Input: dimensioned drawing with shaded views. Units: mm. Origin: part minimum x, y, z. Give positions to 0.01 mm unless a question says otherwise; leave off trailing zeros. Write each loop counter-clockwise with the first axis right and the second up, starting at its lowest first coordinate (ties: lowest second). Pieces come first, ordered by that corner, then holes.
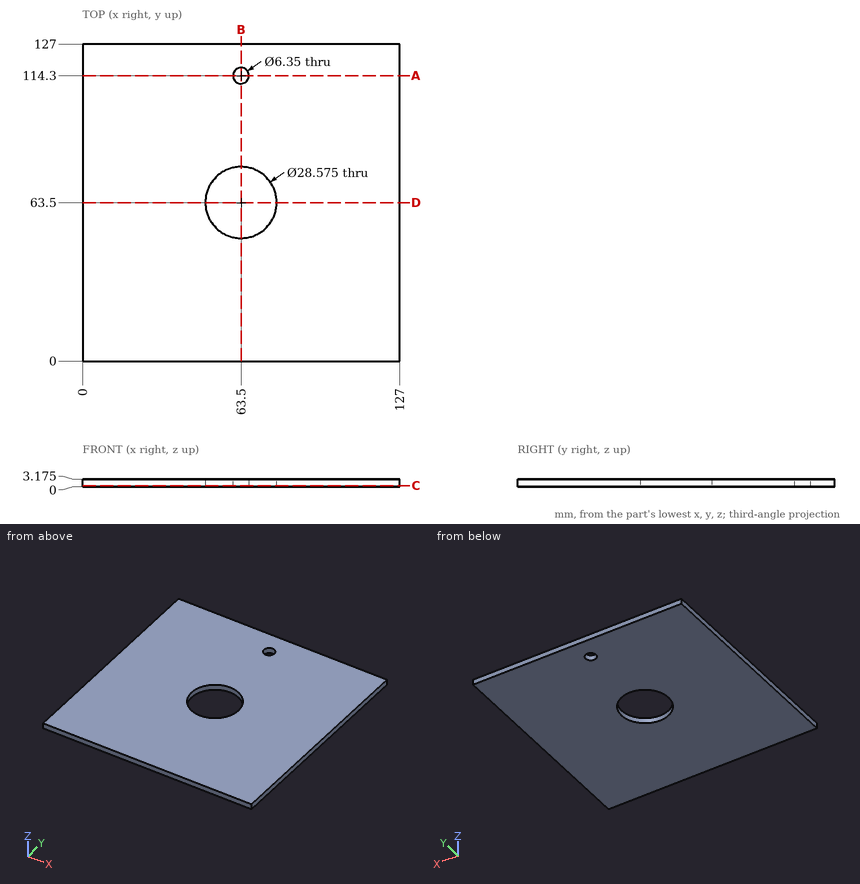
1. Cut plane A-A, the plane y = 114.3. Return the cut outline in (x, z) (3 decimals), then the cut area to 3 significant figures.
2. Cut plane C-C, the plane z = 0.5. State how many separate pieces and enclosed holes the cut face has, then the cut area to 3 significant figures.
3. Contact query for a flat-ended pin moving along its axis: P1, Ø17, axis at x = 63.5, y = 63.5, coming from the +Z side. Output: stop coordinate, or through.
4. Cut plane D-D, the plane y = 63.5. Return the cut outline in (x, z) (1 decimal).
5. Line query: L1, parallel to Y at x = 63.5, z = 1.5 (1 decimal); L2, parallel to X at y = 56, z = 1.2; L3, parallel to X at y = 54.5, z = 0.7. Output: solid intervals per line, ascending.
6. Cut plane B-B, the plane x = 63.5. Return the cut outline in (y, z) (1 decimal).
Response values:
1. outline: (0, 0) - (60.325, 0) - (60.325, 3.175) - (0, 3.175) - close; (66.675, 0) - (127, 0) - (127, 3.175) - (66.675, 3.175) - close
1. area: 383 mm2
2. separate pieces: 1
2. enclosed holes: 2
2. area: 15,500 mm2
3. P1: passes through
4. outline: (0, 0) - (49.2, 0) - (49.2, 3.2) - (0, 3.2) - close; (77.8, 0) - (127, 0) - (127, 3.2) - (77.8, 3.2) - close
5. L1: y = 0 to 49.2, 77.8 to 111.1, 117.5 to 127
5. L2: x = 0 to 51.34, 75.66 to 127
5. L3: x = 0 to 52.4, 74.6 to 127
6. outline: (0, 0) - (49.2, 0) - (49.2, 3.2) - (0, 3.2) - close; (77.8, 0) - (111.1, 0) - (111.1, 3.2) - (77.8, 3.2) - close; (117.5, 0) - (127, 0) - (127, 3.2) - (117.5, 3.2) - close
